```python
from build123d import *

# Parameters (mm, degrees)
SKETCH1_R               = 17.5
BOSS_EXTRUDE1_DEPTH     = 65
SKETCH2_R               = 10
CUT_EXTRUDE1_DEPTH      = 1
CUT_EXTRUDE1_DEPTH_BACK = 66
CHAMFER1_SIZE           = 2.5


with BuildPart() as part:
    # Sketch1 → Boss-Extrude1 (new body)
    with BuildSketch(Plane.XY):
        Circle(SKETCH1_R)
    extrude(amount=BOSS_EXTRUDE1_DEPTH)

    # Sketch2 → Cut-Extrude1 (cut, two sides)
    with BuildSketch(Plane.XY.offset(65)) as cut_extrude1_sk:
        Circle(SKETCH2_R)
    extrude(amount=CUT_EXTRUDE1_DEPTH, mode=Mode.SUBTRACT)
    extrude(cut_extrude1_sk.sketch, amount=-CUT_EXTRUDE1_DEPTH_BACK, mode=Mode.SUBTRACT)

    # Chamfer1
    chamfer1_edges = [part.edges().sort_by_distance(p)[0] for p in [
        (-17.5, 0, 0),
        (-17.5, 0, 65),
    ]]
    chamfer(chamfer1_edges, length=CHAMFER1_SIZE)


solid = part.part
```
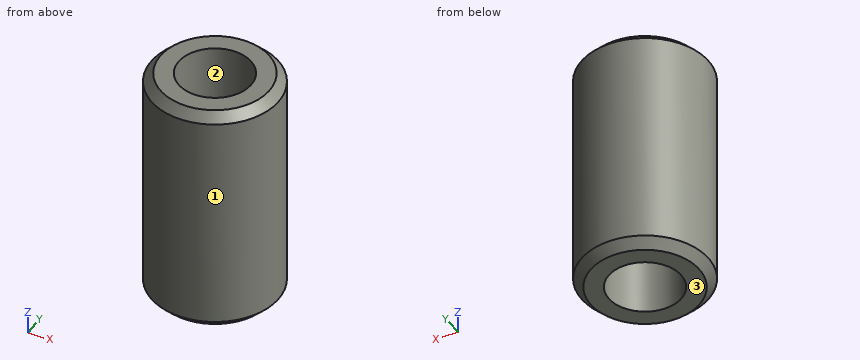
The listing builds one solid part. Answer for the finished solid, in the listing's coordinates (mm). Face numbers are marked on the shaded views. Round coordinates to 2 decimals unless told otherwise and drop trailing zeros. Loops run counter-clockwise (first coordinate to the right, second up) from the corner with the lowest first, then second, coordinate; pieces in that order, holes last.
1) Given P1, Ø12, axis at y = 10, z = 52.5, coming from the -X side; P2, Ø8, axis at y = 12.5, z = 52.5, coming from the -X side; P3, Ø1.5, axis at x = 13, z = 30, coming from the +Y side, each flat-ended and moving along its own axis, determine where each tip first touches the part or whether it passes through.
Outcome:
P1: stops at x = -17.04
P2: stops at x = -15.3
P3: stops at y = 12.5
2) A cutting plane is placed at A-A on x = 0. Determine the outline of the cut face in (y, z), plus the area to 4 significant figures.
Outcome:
outline: (-17.5, 2.5) - (-15, 0) - (-10, 0) - (-10, 65) - (-15, 65) - (-17.5, 62.5) - close; (10, 0) - (15, 0) - (17.5, 2.5) - (17.5, 62.5) - (15, 65) - (10, 65) - close
area: 962.5 mm2
3) A cutting plane is placed at C-C on z = 23. Determine the outline of the cut face in (x, y).
Outcome:
outline: circle Ø35 at (0, 0); hole circle Ø20 at (0, 0)
4) For a pull along Y with two mould halves and no side action, classify the marked faces 1, 2 and 3 as released by +Y, released by -Y, zero draft, split by the parting line, or undercut.
Outcome:
face 1: split by the parting line
face 2: undercut
face 3: zero draft
5) Consider line 1 (Y direction, x = 0, z = 27); line 2 (X direction, y = 9, z = 41.5). Determine where each line is inside the solid, lowest interval first.
Outcome:
line 1: y = -17.5 to -10, 10 to 17.5
line 2: x = -15.01 to -4.36, 4.36 to 15.01
